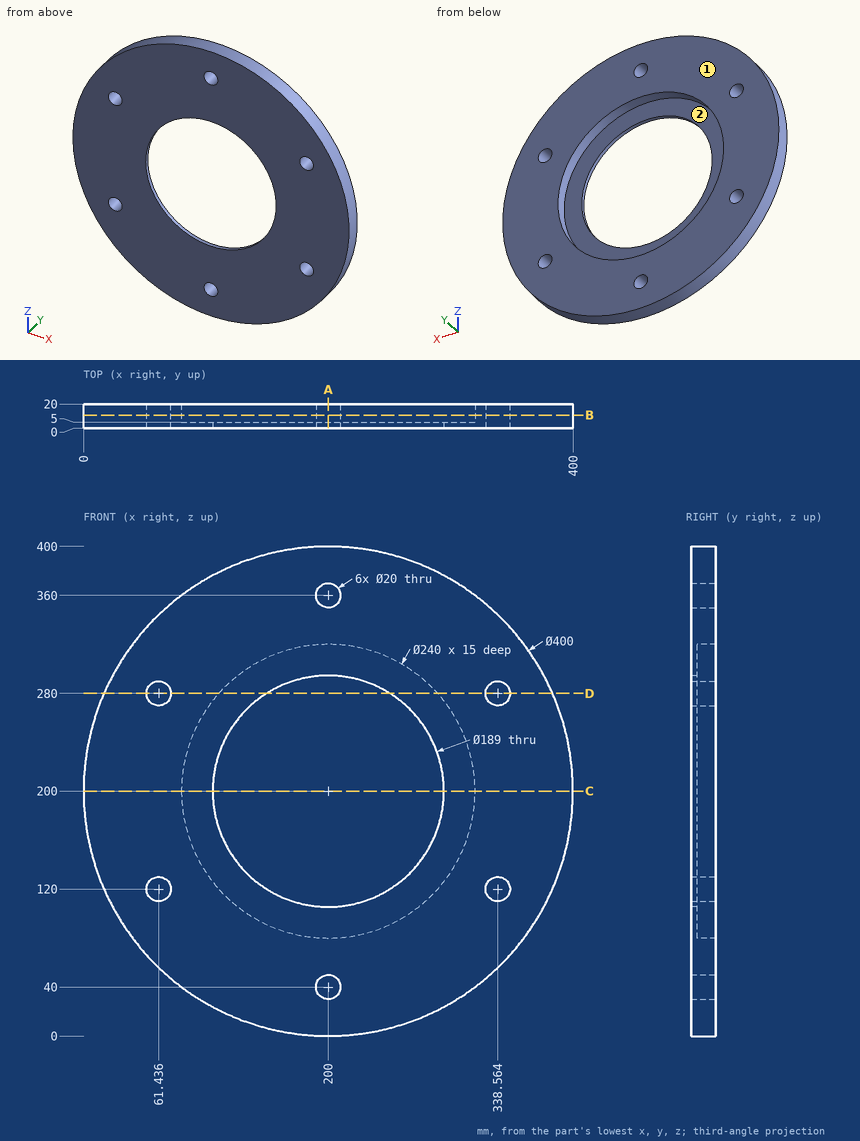
Design review of the part shown in the three views and the two pictorial views. Dimensions are in mm from the part's minimum x, y and z. Coordinates: 2 decimals unless noted, no trailing zeros. Order: outer loops, then holes, each group sorted by start corner. A loop starts at its lowest first (then second) coordinate and runs counter-clockwise, first axis right, second up.
Item 1: For pin 1 Ø3 at (x, y) = (279.5, 12) entering from +Z; pin 2 Ø12 at (x, z) = (312.5, 268) entering from -Y; pin 3 Ø5 at (x, z) = (191.5, 310) entering from +Y; pin 4 Ø6 at (y, z) = (10.5, 107) entering from -X, all flat-tipped, find the tip position at first contact; note any pin that passes through.
Item 2: Take a section at B-B, the plane y = 11. Write out the cut boundary in (x, z), then the cut area to 3 significant figures.
Item 3: Take a section at D-D, the plane z = 280. Write out the cut boundary in (x, y), then the cut area to 3 significant figures.
Item 4: Take a section at A-A, the plane x = 200. Write out the cut boundary in (y, z), then the cut area to 4 significant figures.
Item 5: Take a section at C-C, the plane z = 200. Write out the cut boundary in (x, y).
Item 6: For line 1 (Z direction, x = 200, y = 3.5); line 2 (Z direction, x = 200, y = 14.5); line 3 (X direction, y = 11.25, z = 280), list the stretches that pass through material, from the lowest coordinate up.
Item 7: The part is to be moulded in two halves that separate along Z. For the marked faces 1 and 2, say which applies: pulls with the +Z half, pulls with the -Z half, needs draft (parallel to the pull), parting line crosses it, or undercut.
The answers:
1. pin 1: stops at z = 384.16
1. pin 2: stops at y = 0
1. pin 3: stops at y = 5
1. pin 4: stops at x = 21.39
2. outline: circle Ø400 at (200, 200); hole circle Ø20 at (61.44, 120); hole circle Ø20 at (61.44, 280); hole circle Ø240 at (200, 200); hole circle Ø20 at (200, 40); hole circle Ø20 at (200, 360); hole circle Ø20 at (338.56, 120); hole circle Ø20 at (338.56, 280)
2. area: 78,500 mm2
3. outline: (16.7, 0) - (51.44, 0) - (51.44, 20) - (16.7, 20) - close; (71.44, 0) - (149.7, 0) - (149.7, 5) - (110.56, 5) - (110.56, 20) - (71.44, 20) - close; (250.3, 0) - (328.56, 0) - (328.56, 20) - (289.44, 20) - (289.44, 5) - (250.3, 5) - close; (348.56, 0) - (383.3, 0) - (383.3, 20) - (348.56, 20) - close
3. area: 3,350 mm2
4. outline: (0, 0) - (20, 0) - (20, 30) - (0, 30) - close; (0, 50) - (20, 50) - (20, 80) - (5, 80) - (5, 105.5) - (0, 105.5) - close; (0, 294.5) - (5, 294.5) - (5, 320) - (20, 320) - (20, 350) - (0, 350) - close; (0, 370) - (20, 370) - (20, 400) - (0, 400) - close
4. area: 2,655 mm2
5. outline: (0, 0) - (105.5, 0) - (105.5, 5) - (80, 5) - (80, 20) - (0, 20) - close; (294.5, 0) - (400, 0) - (400, 20) - (320, 20) - (320, 5) - (294.5, 5) - close
6. line 1: z = 0 to 30, 50 to 105.5, 294.5 to 350, 370 to 400
6. line 2: z = 0 to 30, 50 to 80, 320 to 350, 370 to 400
6. line 3: x = 16.7 to 51.44, 71.44 to 110.56, 289.44 to 328.56, 348.56 to 383.3
7. face 1: needs draft
7. face 2: undercut
